Could you check a few things on this model? Use its own coordinates, in mm. A direction names the side the tool comes from. Round coordinates to 2 decimals unless told otherwise and drop trailing zeros. Order: outer loops, then holes, each group sorted by start corner. A loop starts at its lowest first (then second) coordinate and runs counter-clockwise, first axis right, second up. Notation, with made-up numbers: (45, 80) - (100, 80) arc R11 ccw to (100, 94) - close; hole circle Ø5 at (38, -8.5). An arc over 180 degrees is marked (long way). Use one line per item in the form item = value.
from build123d import *

# Parameters (mm, degrees)
SKETCH1_W                                = 60
SKETCH1_H                                = 60
BOSS_EXTRUDE1_DEPTH                      = 5
SKETCH2_R                                = 4
CUT_EXTRUDE1_DEPTH                       = 44.588989435
LPATTERN1_COUNT                          = 3
LPATTERN1_PITCH                          = 15
LPATTERN1_COUNT_DIR2                     = 3
LPATTERN1_PITCH_DIR2                     = 15
CBORE_FOR_M5_PAN_HEAD_SCREW1_D           = 5.5
CBORE_FOR_M5_PAN_HEAD_SCREW1_CBORE_D     = 11
CBORE_FOR_M5_PAN_HEAD_SCREW1_CBORE_DEPTH = 3.7


with BuildPart() as part:
    # Sketch1 → Boss-Extrude1 (new, symmetric)
    with BuildSketch(Plane(origin=(0, 0, 0), x_dir=(0, 1, 0), z_dir=(0, 0, 1))):
        Rectangle(SKETCH1_W, SKETCH1_H)
    extrude(amount=BOSS_EXTRUDE1_DEPTH, both=True)

    # Sketch2 → Cut-Extrude1 (cut, through all)
    with BuildSketch(Plane.XY.offset(5)):
        with Locations((0, -21.213203436)):
            Circle(SKETCH2_R)
    cut_extrude1 = extrude(amount=-CUT_EXTRUDE1_DEPTH, mode=Mode.SUBTRACT)

    # LPattern1: Cut-Extrude1 3 × 3
    with Locations(*[Vector(0.7071067811865476, 0.7071067811865476, 0) * (i * LPATTERN1_PITCH) + Vector(-0.7071067811865476, 0.7071067811865476, 0) * (j * LPATTERN1_PITCH_DIR2) for i in range(LPATTERN1_COUNT) for j in range(LPATTERN1_COUNT_DIR2) if (i, j) != (0, 0)]):
        add(cut_extrude1, mode=Mode.SUBTRACT)

    # CBORE for M5 Pan Head Screw1 (through all)
    with Locations(Plane(origin=(-23, 23, 5), x_dir=(1, 0, 0), z_dir=(0, 0, 1))):
        with Locations((0, 0), (46, 0), (46, -46), (0, -46)):
            CounterBoreHole(CBORE_FOR_M5_PAN_HEAD_SCREW1_D / 2, CBORE_FOR_M5_PAN_HEAD_SCREW1_CBORE_D / 2, CBORE_FOR_M5_PAN_HEAD_SCREW1_CBORE_DEPTH)


solid = part.part
Item 1: Imagine slicing it at D-D on x = -13. Please give me the cut outline in (y, z), plus the area to 3 significant figures.
Found:
outline = (-30, -5) - (-13.81, -5) - (-13.81, 5) - (-30, 5) - close; (-7.4, -5) - (7.4, -5) - (7.4, 5) - (-7.4, 5) - close; (13.81, -5) - (30, -5) - (30, 5) - (13.81, 5) - close
area = 472 mm2
Item 2: Imagine slicing it at B-B on x = 2.5. Please give me the cut outline in (y, z), plus the area to 3 significant figures.
Found:
outline = (-30, -5) - (-24.34, -5) - (-24.34, 5) - (-30, 5) - close; (-18.09, -5) - (-3.12, -5) - (-3.12, 5) - (-18.09, 5) - close; (3.12, -5) - (18.09, -5) - (18.09, 5) - (3.12, 5) - close; (24.34, -5) - (30, -5) - (30, 5) - (24.34, 5) - close
area = 413 mm2
Item 3: If we mould it in two halves opening along Y, with no side actions, what happens to faces 3 (the face through (25.747, 23.121, -1.894)), 4 (the face through (0, -30, 0)), 5 (the face through (-17.754, -21.348, 3.176)), 6 (the face through (30, 0, 0))? For each: released by +Y, released by -Y, zero draft, split by the parting line, or undercut.
Found:
face_3 = undercut
face_4 = released by -Y
face_5 = undercut
face_6 = zero draft
Item 4: I need wall thicknesses on L1, parallel to X at y = 3.5, z = -1.25; L2, parallel to X at y = -14, z = 0.5; L3, parallel to X at y = 0, z = 1.5. Which ranges of each line are inside material? Lowest first, please.
Found:
L1 = -30 to -23.15, -19.28 to -1.94, 1.94 to 19.28, 23.15 to 30
L2 = -30 to -12.72, -8.49 to 8.49, 12.72 to 30
L3 = -30 to -25.21, -17.21 to -4, 4 to 17.21, 25.21 to 30
Item 5: For faces 1 (the face through (-20.253, -22.879, -1.894)), 2 (the face through (20, 22, 1.3)), which set-ups out of +Z, -Z, +X, -X, +Y, -Y let a thin tool reach every point of the face, with its end or its side?
Found:
face_1 = +Z, -Z
face_2 = +Z
Item 6: Will these pins go through, and if not, where does the flat tip stop? P1, Ø10, axis at x = -23, y = -23, coming from the +Z side; P2, Ø6.5, axis at x = -21.21, y = 0, coming from the +Z side.
Found:
P1 = 1.3
P2 = through
Item 7: Imagine slicing it at C-C on z = 2. State how many separate pieces and enclosed holes the cut face has, plus the area to 3 significant figures.
Found:
separate_pieces = 1
enclosed_holes = 13
area = 2,770 mm2
Item 8: Imagine slicing it at A-A on y = 0. Please give me the cut outline in (x, z).
Found:
outline = (-30, -5) - (-25.21, -5) - (-25.21, 5) - (-30, 5) - close; (-17.21, -5) - (-4, -5) - (-4, 5) - (-17.21, 5) - close; (4, -5) - (17.21, -5) - (17.21, 5) - (4, 5) - close; (25.21, -5) - (30, -5) - (30, 5) - (25.21, 5) - close
